from build123d import *

# Parameters (mm, degrees)
SKETCH009_W     = 42
SKETCH009_H     = 42
PAD_DEPTH       = 1.5
POCKET_DEPTH    = 5
SKETCH010_R     = 1.75
POCKET001_DEPTH = 5


with BuildPart() as part:
    # Sketch009 → Pad (new body)
    with BuildSketch(Plane.XY):
        Rectangle(SKETCH009_W, SKETCH009_H)
    extrude(amount=PAD_DEPTH)

    # Sketch (on Face6 of Pad) → Pocket (cut)
    with BuildSketch(Plane.XY.offset(1.5)):
        Polygon((15.08529, 23.560768), (-32.782513, -5.650321), (-32.782513, 34.968018), align=None)
    extrude(amount=-POCKET_DEPTH, mode=Mode.SUBTRACT)

    # Sketch010 (on Face4 of Pocket) → Pocket001 (cut)
    with BuildSketch(Plane.XY.offset(1.5)):
        with Locations((-15.5, 15.5)):
            Circle(SKETCH010_R)
        with Locations((15.5, -15.5)):
            Circle(SKETCH010_R)
        with Locations((15.5, 15.5)):
            Circle(SKETCH010_R)
        with Locations((-15.5, -15.5)):
            Circle(SKETCH010_R)
    extrude(amount=-POCKET001_DEPTH, mode=Mode.SUBTRACT)


solid = part.part
CAD build for the part. Positions are in the model's coordinates, mm. Give positions to 0.01 mm unless a question says otherwise; leave off trailing zeros. Loops run counter-clockwise (first coordinate to the right, second up) from the corner with the lowest first, then second, coordinate; pieces in that order, holes last. Notation, with made-up numbers: M -24,15.5 L 35,15.5 A19 ccw 35,50.5 Z; hole C 60,-24.75 d7. An arc over 180 degrees is marked long. Write each question's results on one line, items separated by ' | '.
Q1. Probe probe 1 along Y at (x, z) = (15.5, 0.85); probe 2 along Y at (x, z) = (-15, 0.2); probe 3 along Y at (x, z) = (-16, 0.85). List the from-to ranges inside material, lowest first.
Geometry check:
probe 1: y = -21 to -17.25, -13.75 to 13.75, 17.25 to 21 | probe 2: y = -21 to -17.18, -13.82 to 5.2 | probe 3: y = -21 to -17.18, -13.82 to 4.59
Q2. Band-saw the part on A-A on x = 15.5. Write the cut outline in (y, z), and give its area (3 significant figures).
Geometry check:
outline: M -21,0 L -17.25,0 L -17.25,1.5 L -21,1.5 Z; M -13.75,0 L 13.75,0 L 13.75,1.5 L -13.75,1.5 Z; M 17.25,0 L 21,0 L 21,1.5 L 17.25,1.5 Z | area: 52.5 mm²
Q3. Mould opens along X. For faces 1 (the face through (0, -4, 1.5)), 2 (the face through (21, 0, 1)), 3 (the face through (-14.6, -14, 0.8)) say: pulls with the +X half, pulls with the -X half, needs draft (parallel to the pull), parting line crosses it, or undercut.
Geometry check:
face 1: needs draft | face 2: pulls with the +X half | face 3: undercut
Q4. Band-saw the part on C-C on z = 0.9. Write the cut outline in (x, y), and give its area (3 significant figures).
Geometry check:
outline: M -21,-21 L 21,-21 L 21,21 L 10.89,21 L -21,1.54 Z; hole C -15.5,-15.5 d3.5; hole C 15.5,-15.5 d3.5; hole C 15.5,15.5 d3.5 | area: 1,420 mm²
Q5. Band-saw the part on D-D on x = -15.5. Write the cut outline in (y, z), and give its area (3 significant figures).
Geometry check:
outline: M -21,0 L -17.25,0 L -17.25,1.5 L -21,1.5 Z; M -13.75,0 L 4.9,0 L 4.9,1.5 L -13.75,1.5 Z | area: 33.6 mm²
